Print and shaded views of the part. All mm, measured from the part's lowest x, y and z. A direction names the side the tool comes from. Round coordinates to 2 decimals unless told otherwise and drop trailing zeros. Order: outer loops, then holes, each group sorted by start corner. A loop starts at its lowest first (then second) coordinate and runs counter-clockwise, first axis right, second up.
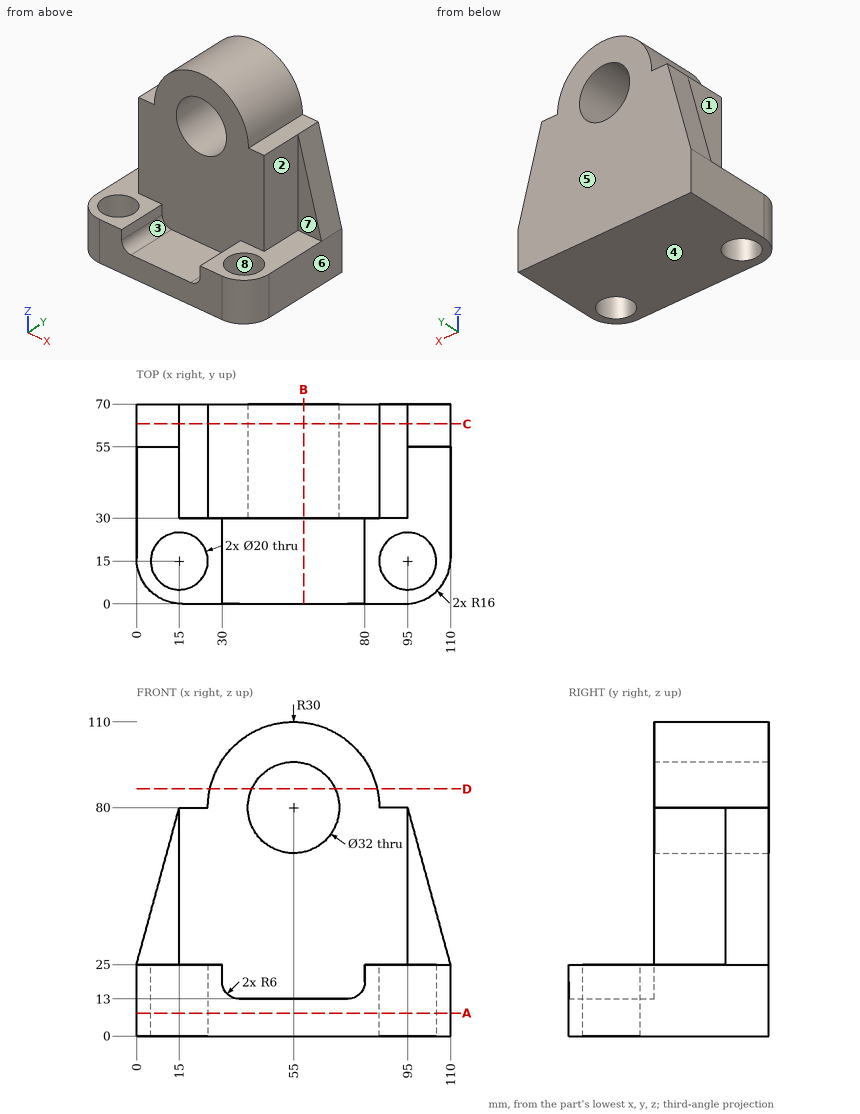
1. Pin check, flat tips, straight feed: P1, Ø4, axis at x = 58.5, z = 46.5, coming from the -Y side; P2, Ø6, axis at y = 42.5, z = 70.5, coming from the +X side; P3, Ø7.5, axis at y = 38.5, z = 53, coming from the -X side. Stop position of each tip, or through.
2. Drill centre lines: line 1 (Y direction, x = 15, z = 17); line 2 (Z direction, x = 56, y = 38); line 3 (X direction, y = 13, z = 8.5). Where is each one in solid material? Low to high.
3. Mould opens along Y. For the marked faces 5, 6, 7 and 8 say: released by +Y, released by -Y, zero draft, split by the parting line, or undercut.
4. Cut at A-A, the plane z = 8. Write the cut outline in (x, y).
5. Tool access for the marked faces 1, 2, 3 and 4: list every direction of +Z, -Z, +X, -X, +Y, -Y with a clear straight run to the whole face (end or side of a thin tool).
6. Cut at C-C, the plane y = 63. Write the cut outline in (x, z).
7. Cut at B-B, the plane x = 58.5. Write the cut outline in (y, z).
8. Cut at D-D, the plane z = 86.5. Write the cut outline in (x, y).
Outcome:
1. P1: stops at y = 30
1. P2: stops at x = 95
1. P3: stops at x = 15
2. line 1: y = 0.03 to 5, 25 to 70
2. line 2: z = 0 to 64.03, 95.97 to 109.98
2. line 3: x = 0.28 to 5.2, 24.8 to 85.2, 104.8 to 109.72
3. face 5: released by +Y
3. face 6: zero draft
3. face 7: released by -Y
3. face 8: undercut
4. outline: (0, 16) arc R16 ccw to (16, 0) - (94, 0) arc R16 ccw to (110, 16) - (110, 70) - (0, 70) - close; hole circle Ø20 at (15, 15); hole circle Ø20 at (95, 15)
5. face 1: +Z, -X, -Y
5. face 2: +Z, +X, -Y
5. face 3: +Z, -Y
5. face 4: -Z, +X, -X, +Y, -Y
6. outline: (0, 0) - (110, 0) - (110, 25) - (95, 80) - (85, 80) arc R30 ccw to (25, 80) - (15, 80) - (0, 25) - close; hole circle Ø32 at (55, 80)
7. outline: (0, 0) - (70, 0) - (70, 64.39) - (30, 64.39) - (30, 13) - (0, 13) - close; (30, 95.61) - (70, 95.61) - (70, 109.8) - (30, 109.8) - close
8. outline: (25.71, 30) - (40.38, 30) - (40.38, 70) - (25.71, 70) - close; (69.62, 30) - (84.29, 30) - (84.29, 70) - (69.62, 70) - close
